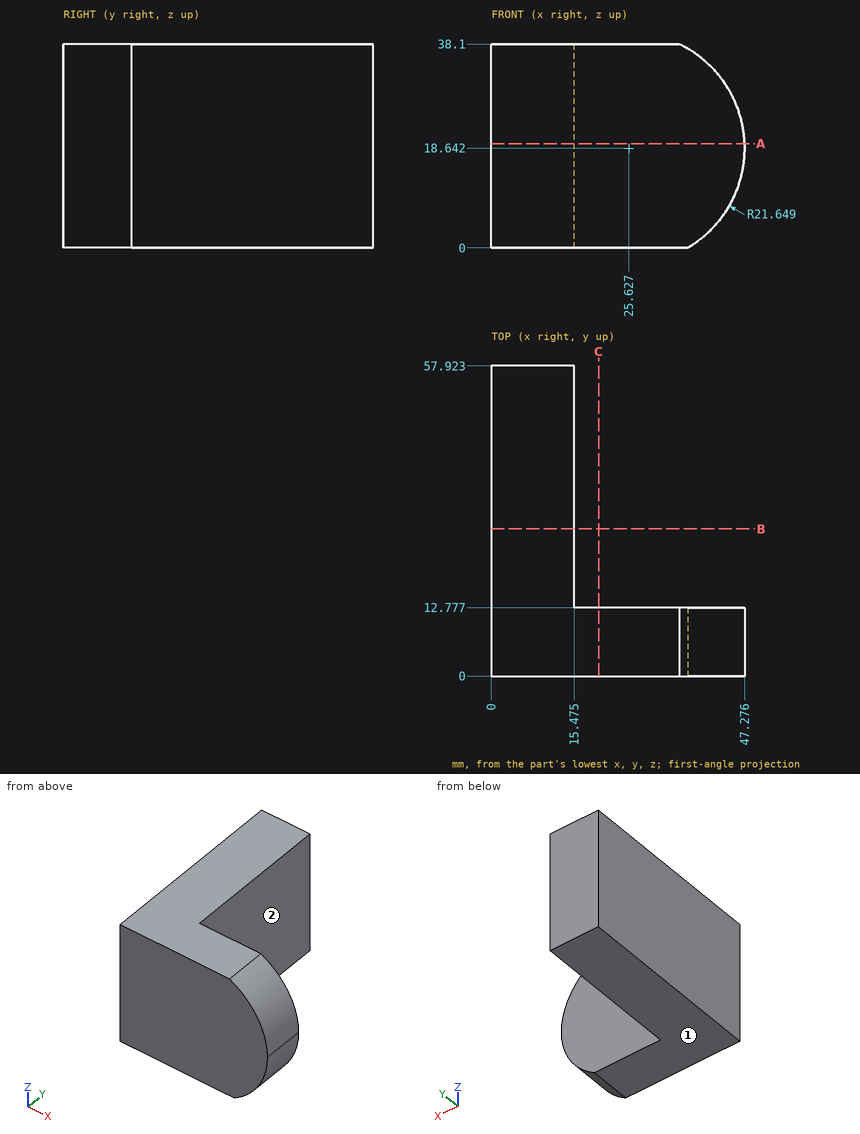
Drawing for the job (mm, zero at the part's lowest x, y, z). A direction names the side the tool comes from. Round coordinates to 2 decimals unless told otherwise and drop trailing zeros. Loops run counter-clockwise (first coordinate to the right, second up) from the corner with the lowest first, then second, coordinate; pieces in that order, holes last.
1. Band-saw the part on C-C, the plane x = 20. List the corners of the cut face in (y, z), and give its area (3 significant figures).
Check values:
outline: (0, 0) - (12.78, 0) - (12.78, 38.1) - (0, 38.1) - close
area: 487 mm2
2. Band-saw the part on B-B, the plane y = 27.5. List the corners of the cut face in (x, z) (1 decimal).
Check values:
outline: (0, 0) - (15.5, 0) - (15.5, 38.1) - (0, 38.1) - close
3. Wall check: probe 1 along X at (y, z) = (42.5, 15.5) (1 decimal); probe 2 along Y at (x, z) = (31.5, 35); probe 3 along X at (y, z) = (6, 33.5). Give the ranges that are in metal, low to high.
Check values:
probe 1: x = 0 to 15.5
probe 2: y = 0 to 12.78
probe 3: x = 0 to 41.37
4. Band-saw the part on A-A, the plane z = 19.5. List the corners of the cut face in (x, y) (1 decimal).
Check values:
outline: (0, 0) - (47.3, 0) - (47.3, 12.8) - (15.5, 12.8) - (15.5, 57.9) - (0, 57.9) - close
5. Drop flat-ended pins along their axis: P1, Ø6, axis at y = 20.5, z = 25, coming from the +X side (1 decimal); P2, Ø16, axis at x = 31.5, z = 13, coming from the +Y side. Give the stop position or say it passes through.
Check values:
P1: stops at x = 15.5
P2: stops at y = 12.78
6. Tool access for the marked faces 1 and 2: list every direction of +Z, -Z, +X, -X, +Y, -Y with a clear straight run to the whole face (end or side of a thin tool).
Check values:
face 1: -Z, +X, -X, +Y, -Y
face 2: +Z, -Z, +X, +Y
